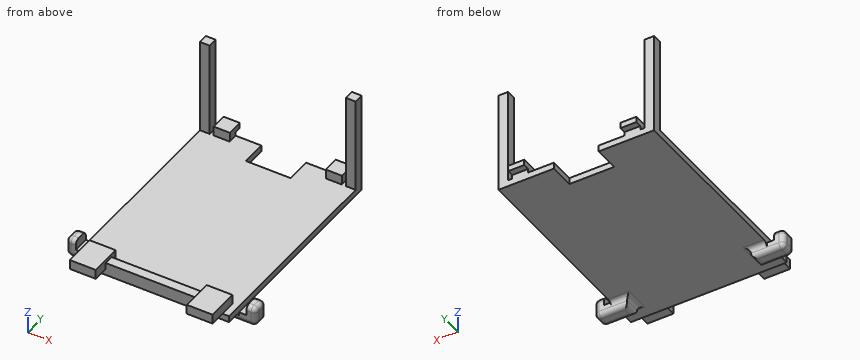
```python
from build123d import *

# Parameters (mm, degrees)
SKETCH_1_W             = 48.6
SKETCH_1_H             = 66.8
EXTRUDE_1_DEPTH        = 2
SKETCH_2_W             = 8.1
SKETCH_2_H             = 10
EXTRUDE_2_DEPTH        = 3
SKETCH_3_W             = 28.4
SKETCH_3_H             = 3
EXTRUDE_3_DEPTH        = 2
SKETCH_4_W             = 14
SKETCH_4_H             = 8
CUT_EXTRUDE_1_DEPTH    = 88.976587795
SKETCH_5_W             = 5
SKETCH_5_H             = 5
EXTRUDE_4_DEPTH        = 3
SKETCH_6_W             = 5
SKETCH_6_H             = 1.2
CUT_EXTRUDE_2_DEPTH    = 2
SKETCH_7_W             = 3
SKETCH_7_H             = 3
EXTRUDE_5_DEPTH        = 29.8
SKETCH_8_W             = 10.3
SKETCH_8_H             = 5
EXTRUDE_6_DEPTH        = 3
SKETCH_9_W             = 3
SKETCH_9_H             = 5
EXTRUDE_7_DEPTH        = 3
FILLET_1_R             = 1.5
FILLET_1_OF_MIRROR_2_R = 1.5


with BuildPart() as part:
    # 草图1 → 凸台-拉伸1 (new body)
    with BuildSketch(Plane(origin=(0, 0, -32), x_dir=(-1, 0, 0), z_dir=(0, 0, -1))):
        with Locations((-14.5, 45.4)):
            Rectangle(SKETCH_1_W, SKETCH_1_H)
    extrude(amount=-EXTRUDE_1_DEPTH)

    # 草图2 → 凸台-拉伸2 (add)
    with BuildSketch(Plane.XY.offset(-30)):
        with Locations((-3.75, 12)):
            Rectangle(SKETCH_2_W, SKETCH_2_H)
    extrude_2 = extrude(amount=EXTRUDE_2_DEPTH)

    # 镜向1: 凸台-拉伸2 across plane
    add(extrude_2.mirror(Plane.ZY.offset(-14.5)))

    # 草图3 → 凸台-拉伸3 (add)
    with BuildSketch(Plane.XY.offset(-30)):
        with Locations((14.5, 13.5)):
            Rectangle(SKETCH_3_W, SKETCH_3_H)
    extrude(amount=EXTRUDE_3_DEPTH)

    # 草图4 → 切除-拉伸1 (cut, through all)
    with BuildSketch(Plane(origin=(0, 0, -32), x_dir=(-1, 0, 0), z_dir=(0, 0, -1))):
        with Locations((-14.5, 75)):
            Rectangle(SKETCH_4_W, SKETCH_4_H)
    extrude(amount=-CUT_EXTRUDE_1_DEPTH, mode=Mode.SUBTRACT)

    # 草图5 → 凸台-拉伸4 (add)
    with BuildSketch(Plane.XY.offset(-30)):
        with Locations((-3, 78.3)):
            Rectangle(SKETCH_5_W, SKETCH_5_H)
        with Locations((32, 78.3)):
            Rectangle(SKETCH_5_W, SKETCH_5_H)
    extrude(amount=EXTRUDE_4_DEPTH)

    # 草图6 → 切除-拉伸2 (cut)
    with BuildSketch(Plane(origin=(0, 80.8, 0), x_dir=(1, 0, 0), z_dir=(0, 1, 0))):
        with Locations((-3, 29.4)):
            Rectangle(SKETCH_6_W, SKETCH_6_H)
        with Locations((32, 29.4)):
            Rectangle(SKETCH_6_W, SKETCH_6_H)
    extrude(amount=-CUT_EXTRUDE_2_DEPTH, mode=Mode.SUBTRACT)

    # 草图7 → 凸台-拉伸5 (add)
    with BuildSketch(Plane.XY.offset(-30)):
        with Locations((-8.3, 77.3)):
            Rectangle(SKETCH_7_W, SKETCH_7_H)
        with Locations((37.3, 77.3)):
            Rectangle(SKETCH_7_W, SKETCH_7_H)
    extrude(amount=EXTRUDE_5_DEPTH)

    # 草图8 → 凸台-拉伸6 (add)
    with BuildSketch(Plane(origin=(0, 0, -32), x_dir=(-1, 0, 0), z_dir=(0, 0, -1))):
        with Locations((9.95, 19.5)):
            Rectangle(SKETCH_8_W, SKETCH_8_H)
    extrude_6 = extrude(amount=EXTRUDE_6_DEPTH)

    # 草图9 → 凸台-拉伸7 (add)
    with BuildSketch(Plane.XY.offset(-32)):
        with Locations((-13.6, 19.5)):
            Rectangle(SKETCH_9_W, SKETCH_9_H)
    extrude_7 = extrude(amount=EXTRUDE_7_DEPTH)

    # 圆角1
    fillet_1_edges = [part.edges().sort_by_distance(p)[0] for p in [
        (-15.1, 19.5, -29),
        (-15.1, 22, -32),
        (-15.1, 17, -32),
        (-4.8, 19.5, -32),
        (-7.3, 17, -32),
        (-9.95, 17, -35),
        (-4.8, 19.5, -35),
        (-7.3, 22, -32),
        (-9.95, 22, -35),
        (-15.1, 19.5, -35),
        (-13.6, 22, -29),
        (-13.6, 17, -29),
    ]]
    fillet(fillet_1_edges, radius=FILLET_1_R - 0.0001)  # a hair under: the kernel refuses the full size

    # 镜向2: 凸台-拉伸6, 凸台-拉伸7 across plane
    add(extrude_6.mirror(Plane.ZY.offset(-14.5)))
    add(extrude_7.mirror(Plane.ZY.offset(-14.5)))

    # 圆角1 of 镜向2
    fillet_1_of_mirror_2_edges = [part.edges().sort_by_distance(p)[0] for p in [
        (44.1, 19.5, -29),
        (44.1, 22, -32),
        (44.1, 17, -32),
        (33.8, 19.5, -32),
        (36.3, 17, -32),
        (38.95, 17, -35),
        (33.8, 19.5, -35),
        (36.3, 22, -32),
        (38.95, 22, -35),
        (44.1, 19.5, -35),
        (42.6, 22, -29),
        (42.6, 17, -29),
    ]]
    fillet(fillet_1_of_mirror_2_edges, radius=FILLET_1_OF_MIRROR_2_R - 0.0001)  # a hair under: the kernel refuses the full size


solid = part.part
```
Model file for the job. Use its own axes, mm. Coordinates: 2 decimals unless noted, no trailing zeros. Order: outer loops, then holes, each group sorted by start corner. A loop starts at its lowest first (then second) coordinate and runs counter-clockwise, first axis right, second up. Notation, with made-up numbers: (35, 77.5) - (84, 77.5) arc R26 cw to (84, 104.5) - close; hole circle Ø6 at (85.25, -19). An arc over 180 degrees is marked (long way). Return JSON: item names as keys, results as strings. Group by question number.
1) Saw through at D-D, the plane y = 69. Write the cut outline in (x, z), plus the area to 3 significant figures.
2) Probe line 1 (Y direction, x = 30, z = -29.5); line 2 (Y direction, x = 32, z = -28); line 3 (Z direction, x = -8.5, y = 68). List the from-to ranges inside material, lowest first. Write a range as from..to.
3) Flat gauge pins, fed straight in: P1, Ø0.8, axis at x = -13, y = 19.5, coming from the +Z side; P2, Ø12, axis at x = 26, y = 38, coming from the +Z side; P3, Ø1.5, axis at x = 12, y = 13.5, coming from the +Z side. Where does each tip first touch, or does it go through?
4) Saw through at A-A, the plane z = -21.5. Write the cut outline in (x, y).
5) Saw through at C-C, the plane x = 11. Write the cut outline in (y, z).
Values found:
{
 "1": {"outline": "(-9.8, -32) - (38.8, -32) - (38.8, -30) - (-9.8, -30) - close", "area": "97.2 mm²"},
 "2": {"line 1": "y = 7..17, 75.8..78.8", "line 2": "y = 7..17, 75.8..80.8", "line 3": "z = -32..-30"},
 "3": {"P1": "stops at z = -29", "P2": "stops at z = -30", "P3": "stops at z = -28"},
 "4": {"outline": "(-9.8, 75.8) - (-6.8, 75.8) - (-6.8, 78.8) - (-9.8, 78.8) - close; (35.8, 75.8) - (38.8, 75.8) - (38.8, 78.8) - (35.8, 78.8) - close"},
 "5": {"outline": "(12, -32) - (71, -32) - (71, -30) - (15, -30) - (15, -28) - (12, -28) - close"}
}
